Read the model definition and answer for the solid it produces. Units are mm, in the model's axes. A direction names the side the tool comes from. Coordinates: 2 decimals unless noted, no trailing zeros. Loops run counter-clockwise (first coordinate to the right, second up) from the corner with the lowest first, then second, coordinate; pieces in that order, holes last. Notation, with made-up numbers: M 17,-10.5 L 57,-10.5 A25 cw 57,19.5 Z; hole C 52.5,63 d4. An arc over 180 degrees is marked long. One line per item, written item: value. Start each with the question number.
1. For faces 1 (the face through (-64, 96, 2)), 2 (the face through (-213.289, 5.539, 2.125)), determine the directions among +Z, -Z, +X, -X, +Y, -Y from which every point of the face is accessible in a straight line to the end or side of a thin tool.
2. Flat-ended cylindrical pins translate along their axes: pin 1 (4 mm diameter, centred on x = -215, y = 84, fed in from +Z); pin 2 (4.5 mm diameter, centred on x = -159, y = 3, fed in from +Z); pin 3 (2 mm diameter, centred on x = -159, y = 164, fed in from -Z); pin 4 (1.2 mm diameter, centred on x = -113, z = 3, fed in from -Y). Find the tip coordinate at first contact, or state that the pin passes through.
3. The part is cut by section B-B (x = -195.5). Write down the section's boundary in (y, z).
4. The part is cut by section C-C (y = 30). Write down the section's boundary in (x, z), then the cut area to 3 significant figures.
5. Consider probe 1 along X at (y, z) = (102, 2.8); probe 2 along Y at (x, z) = (-59, 1.2); probe 3 along Y at (x, z) = (-3, 1). Determine where each line is inside the solid, lowest interval first.
6. The part is cut by section A-A (y = 66). Write down the section's boundary in (x, z).
7. The part is cut by section D-D (x = -79.5). State how many separate pieces and enclosed holes the cut face has, then the cut area to 3 significant figures.
```python
from build123d import *

# Parameters (mm, degrees)
SKETCH1_W           = 168
SKETCH1_H           = 218
SKETCH1_R           = 1.7
BOSS_EXTRUDE2_DEPTH = 4
CHAMFER1_SIZE       = 2
CHAMFER1_SIZE_2     = 1.5
FILLET1_R           = 2


with BuildPart() as part:
    # Sketch1 → Boss-Extrude2 (new body)
    with BuildSketch(Plane(origin=(0, 0, 0), x_dir=(0, 1, 0), z_dir=(0, 0, 1))):
        with Locations((84, 109)):
            Rectangle(SKETCH1_W, SKETCH1_H)
        with Locations(Location((5, 3, 0), (0, 0, 270))):
            Circle(SKETCH1_R, mode=Mode.SUBTRACT)
        with Locations(Location((5, 215, 0), (0, 0, 270))):
            Circle(SKETCH1_R, mode=Mode.SUBTRACT)
        with Locations(Location((163, 215, 0), (0, 0, 270))):
            Circle(SKETCH1_R, mode=Mode.SUBTRACT)
        with Locations(Location((163, 3, 0), (0, 0, 270))):
            Circle(SKETCH1_R, mode=Mode.SUBTRACT)
        with Locations(Location((84, 215, 0), (0, 0, 270))):
            Circle(SKETCH1_R, mode=Mode.SUBTRACT)
        with Locations(Location((84, 3, 0), (0, 0, 270))):
            Circle(SKETCH1_R, mode=Mode.SUBTRACT)
        with Locations(Location((3, 59, 0), (0, 0, 270))):
            Circle(SKETCH1_R, mode=Mode.SUBTRACT)
        with Locations(Location((164, 59, 0), (0, 0, 270))):
            Circle(SKETCH1_R, mode=Mode.SUBTRACT)
        with Locations(Location((164, 159, 0), (0, 0, 270))):
            Circle(SKETCH1_R, mode=Mode.SUBTRACT)
        with Locations(Location((3, 159, 0), (0, 0, 270))):
            Circle(SKETCH1_R, mode=Mode.SUBTRACT)
        with BuildLine():
            Line((35, 149), (35, 69))
            ThreePointArc((35, 69), (30, 64), (25, 69))
            Line((25, 69), (25, 149))
            ThreePointArc((25, 149), (30, 154), (35, 149))
        make_face(mode=Mode.SUBTRACT)
        with BuildLine():
            Line((57, 149), (57, 69))
            ThreePointArc((57, 69), (52, 64), (47, 69))
            Line((47, 69), (47, 149))
            ThreePointArc((47, 149), (52, 154), (57, 149))
        make_face(mode=Mode.SUBTRACT)
        with BuildLine():
            Line((79, 149), (79, 69))
            ThreePointArc((79, 69), (74, 64), (69, 69))
            Line((69, 69), (69, 149))
            ThreePointArc((69, 149), (74, 154), (79, 149))
        make_face(mode=Mode.SUBTRACT)
        with BuildLine():
            Line((101, 149), (101, 69))
            ThreePointArc((101, 69), (96, 64), (91, 69))
            Line((91, 69), (91, 149))
            ThreePointArc((91, 149), (96, 154), (101, 149))
        make_face(mode=Mode.SUBTRACT)
        with BuildLine():
            Line((123, 149), (123, 69))
            ThreePointArc((123, 69), (118, 64), (113, 69))
            Line((113, 69), (113, 149))
            ThreePointArc((113, 149), (118, 154), (123, 149))
        make_face(mode=Mode.SUBTRACT)
        with BuildLine():
            Line((145, 149), (145, 69))
            ThreePointArc((145, 69), (140, 64), (135, 69))
            Line((135, 69), (135, 149))
            ThreePointArc((135, 149), (140, 154), (145, 149))
        make_face(mode=Mode.SUBTRACT)
        with BuildLine():
            Line((25, 208), (143, 208))
            ThreePointArc((143, 208), (155.5, 195.5), (143, 183))
            Line((143, 183), (25, 183))
            ThreePointArc((25, 183), (12.5, 195.5), (25, 208))
        make_face(mode=Mode.SUBTRACT)
        with BuildLine():
            Line((25, 35), (143, 35))
            ThreePointArc((143, 35), (155.5, 22.5), (143, 10))
            Line((143, 10), (25, 10))
            ThreePointArc((25, 10), (12.5, 22.5), (25, 35))
        make_face(mode=Mode.SUBTRACT)
    extrude(amount=BOSS_EXTRUDE2_DEPTH)

    # Chamfer1
    # the kernel refuses this chamfer: 2, 1.5 mm, written as the material it takes off along each edge
    with BuildSketch(Plane(origin=(-3, 5, 4), x_dir=(1, 0, 0), z_dir=(0, -1, 0))) as chamfer1_piece_1:
        Polygon((1.7, -CHAMFER1_SIZE), (1.7 + CHAMFER1_SIZE_2, 0), (1.7, 0), align=None)
    revolve(axis=Axis((-3, 5, 4), (0, 0, 1)), mode=Mode.SUBTRACT)
    with BuildSketch(Plane(origin=(-59, 3, 4), x_dir=(1, 0, 0), z_dir=(0, -1, 0))) as chamfer1_piece_2:
        Polygon((1.7, -CHAMFER1_SIZE), (1.7 + CHAMFER1_SIZE_2, 0), (1.7, 0), align=None)
    revolve(axis=Axis((-59, 3, 4), (0, 0, 1)), mode=Mode.SUBTRACT)
    with BuildSketch(Plane(origin=(-59, 164, 4), x_dir=(1, 0, 0), z_dir=(0, -1, 0))) as chamfer1_piece_3:
        Polygon((1.7, -CHAMFER1_SIZE), (1.7 + CHAMFER1_SIZE_2, 0), (1.7, 0), align=None)
    revolve(axis=Axis((-59, 164, 4), (0, 0, 1)), mode=Mode.SUBTRACT)
    with BuildSketch(Plane(origin=(-159, 164, 4), x_dir=(1, 0, 0), z_dir=(0, -1, 0))) as chamfer1_piece_4:
        Polygon((1.7, -CHAMFER1_SIZE), (1.7 + CHAMFER1_SIZE_2, 0), (1.7, 0), align=None)
    revolve(axis=Axis((-159, 164, 4), (0, 0, 1)), mode=Mode.SUBTRACT)
    with BuildSketch(Plane(origin=(-159, 3, 4), x_dir=(1, 0, 0), z_dir=(0, -1, 0))) as chamfer1_piece_5:
        Polygon((1.7, -CHAMFER1_SIZE), (1.7 + CHAMFER1_SIZE_2, 0), (1.7, 0), align=None)
    revolve(axis=Axis((-159, 3, 4), (0, 0, 1)), mode=Mode.SUBTRACT)
    with BuildSketch(Plane(origin=(-215, 5, 4), x_dir=(1, 0, 0), z_dir=(0, -1, 0))) as chamfer1_piece_6:
        Polygon((1.7, -CHAMFER1_SIZE), (1.7 + CHAMFER1_SIZE_2, 0), (1.7, 0), align=None)
    revolve(axis=Axis((-215, 5, 4), (0, 0, 1)), mode=Mode.SUBTRACT)
    with BuildSketch(Plane(origin=(-215, 163, 4), x_dir=(1, 0, 0), z_dir=(0, -1, 0))) as chamfer1_piece_7:
        Polygon((1.7, -CHAMFER1_SIZE), (1.7 + CHAMFER1_SIZE_2, 0), (1.7, 0), align=None)
    revolve(axis=Axis((-215, 163, 4), (0, 0, 1)), mode=Mode.SUBTRACT)
    with BuildSketch(Plane(origin=(-3, 163, 4), x_dir=(1, 0, 0), z_dir=(0, -1, 0))) as chamfer1_piece_8:
        Polygon((1.7, -CHAMFER1_SIZE), (1.7 + CHAMFER1_SIZE_2, 0), (1.7, 0), align=None)
    revolve(axis=Axis((-3, 163, 4), (0, 0, 1)), mode=Mode.SUBTRACT)
    with BuildSketch(Plane(origin=(-215, 84, 4), x_dir=(1, 0, 0), z_dir=(0, -1, 0))) as chamfer1_piece_9:
        Polygon((1.7, -CHAMFER1_SIZE), (1.7 + CHAMFER1_SIZE_2, 0), (1.7, 0), align=None)
    revolve(axis=Axis((-215, 84, 4), (0, 0, 1)), mode=Mode.SUBTRACT)
    with BuildSketch(Plane(origin=(-3, 84, 4), x_dir=(1, 0, 0), z_dir=(0, -1, 0))) as chamfer1_piece_10:
        Polygon((1.7, -CHAMFER1_SIZE), (1.7 + CHAMFER1_SIZE_2, 0), (1.7, 0), align=None)
    revolve(axis=Axis((-3, 84, 4), (0, 0, 1)), mode=Mode.SUBTRACT)

    # Fillet1
    # the kernel refuses this fillet: 2 mm, written as the material it takes off along each edge
    with BuildSketch(Plane(origin=(5, 168, 4), x_dir=(0, 0, -1), z_dir=(-1, 0, 0))) as fillet1_piece_1:
        with BuildLine():
            CenterArc((FILLET1_R, FILLET1_R), FILLET1_R, 180, 90)
            Line((0, FILLET1_R), (0, 0))
            Line((0, 0), (FILLET1_R, 0))
        make_face()
    extrude(amount=228, mode=Mode.SUBTRACT)
    with BuildSketch(Plane(origin=(-162.886447127, 0, 4), x_dir=(0, 1, 0), z_dir=(1, 0, 0))) as fillet1_piece_2:
        with BuildLine():
            CenterArc((FILLET1_R, -FILLET1_R), FILLET1_R, 90, 90)
            Line((0, -FILLET1_R), (0, 0))
            Line((0, 0), (FILLET1_R, 0))
        make_face()
    extrude(amount=107.772894255, mode=Mode.SUBTRACT)
    with BuildSketch(Plane(origin=(-62.886447127, 0, 4), x_dir=(0, 1, 0), z_dir=(1, 0, 0)), Plane(origin=(-223, 0, 4), x_dir=(0, 1, 0), z_dir=(1, 0, 0))) as fillet1_piece_3:
        with BuildLine():
            CenterArc((FILLET1_R, -FILLET1_R), FILLET1_R, 90, 90)
            Line((0, -FILLET1_R), (0, 0))
            Line((0, 0), (FILLET1_R, 0))
        make_face()
    extrude(amount=67.886447127, mode=Mode.SUBTRACT)


solid = part.part
```
Answer block:
1. face 1: +Z, -Z
1. face 2: +Z
2. pin 1: stops at z = 2.4
2. pin 2: stops at z = 2.73
2. pin 3: passes through
2. pin 4: stops at y = 0.04
3. outline: M 0,0 L 12.5,0 L 12.5,4 L 2,4 A2 ccw 0,2 Z; M 155.5,0 L 168,0 L 168,2 A2 ccw 166,4 L 155.5,4 Z
4. outline: M -218,0 L -208,0 L -208,4 L -218,4 Z; M -183,0 L -154,0 L -154,4 L -183,4 Z; M -64,0 L -35,0 L -35,4 L -64,4 Z; M -10,0 L 0,0 L 0,4 L -10,4 Z
4. area: 312 mm2
5. probe 1: x = -218 to -208, -183 to -35, -10 to 0
5. probe 2: y = 0 to 1.3, 4.7 to 162.3, 165.7 to 168
5. probe 3: y = 0 to 3.3, 6.7 to 82.3, 85.7 to 161.3, 164.7 to 168
6. outline: M -218,0 L -208,0 L -208,4 L -218,4 Z; M -183,0 L -35,0 L -35,4 L -183,4 Z; M -10,0 L 0,0 L 0,4 L -10,4 Z
7. separate pieces: 7
7. enclosed holes: 0
7. area: 430 mm2
